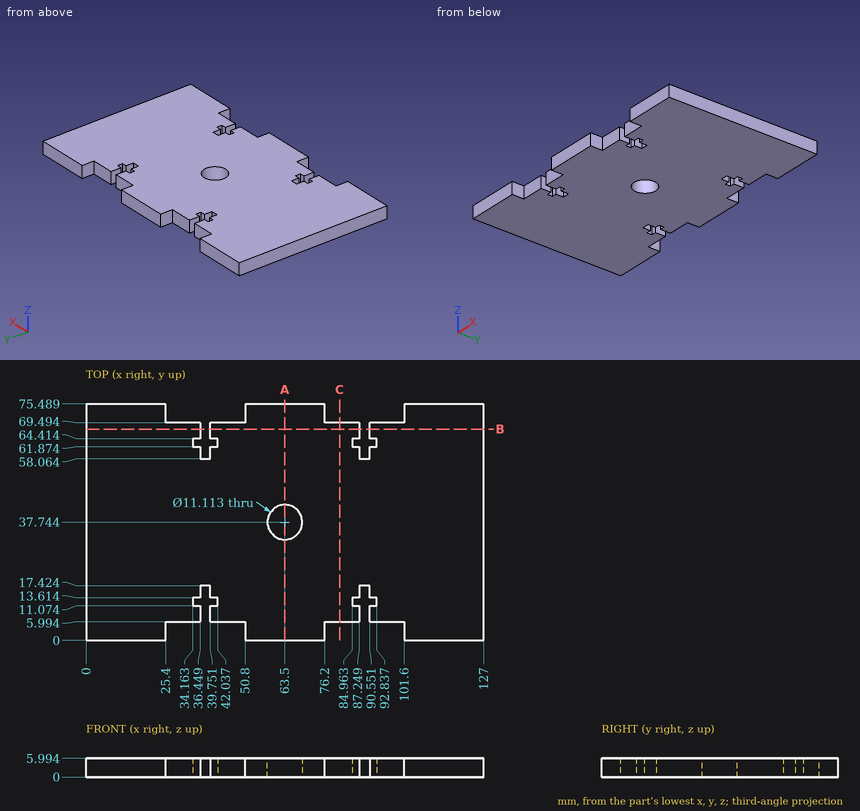
Print and shaded views of the part. All mm, measured from the part's lowest x, y and z. Round coordinates to 2 decimals unless told otherwise and drop trailing zeros. Write each loop counter-clockwise with the first axis right and the second up, starting at its lowest first coordinate (ties: lowest second). Pieces come first, ordered by that corner, then holes.
(1) Drop flat-ended pins along their axis: P1, Ø1.8, axis at x = 92, z = 2, coming from the -Y side; P2, Ø1.8, axis at x = 35, z = 3.5, coming from the +Y side. Give the stop position or say it passes through.
(2) Probe line 1 along X through (y, z) = (5, 1.8); line 2 along Y through (x, z) = (36, 4.6) (1 decimal); line 3 along X through (y, z) = (66.5, 2.2). List the from-to ranges inside material, lowest first.
(3) Slice it at C-C, the plane x = 81. Write the cut outline in (y, z) (1 decimal), and give its area (3 significant figures).
(4) Slice it at A-A, the plane x = 63.5. Write the cut outline in (y, z) (1 decimal).
(5) Slice it at B-B, the plane y = 67.5. Count the separate pieces of the cut face and the enclosed holes in it.
From the geometry:
1. P1: stops at y = 5.99
1. P2: stops at y = 69.49
2. line 1: x = 0 to 25.4, 50.8 to 76.2, 101.6 to 127
2. line 2: y = 6 to 11.1, 13.6 to 61.9, 64.4 to 69.5
2. line 3: x = 0 to 36.45, 39.75 to 87.25, 90.55 to 127
3. outline: (6, 0) - (69.5, 0) - (69.5, 6) - (6, 6) - close
3. area: 381 mm2
4. outline: (0, 0) - (32.2, 0) - (32.2, 6) - (0, 6) - close; (43.3, 0) - (75.5, 0) - (75.5, 6) - (43.3, 6) - close
5. separate pieces: 3
5. enclosed holes: 0
